from build123d import *

# Parameters (mm, degrees)
CROQUIS1_R                 = 2
SALIENTE_EXTRUIR1_DEPTH    = 16.65
CORTAR_EXTRUIR1_DEPTH      = 12.5
CORTAR_EXTRUIR1_DEPTH_BACK = 12.5
CROQUIS2_R                 = 2
CROQUIS2_R_2               = 1.505
REDONDEO1_R                = 0.5
REDONDEO2_R                = 0.5


with BuildPart() as part:
    # Croquis1 → Saliente-Extruir1 (new, symmetric)
    with BuildSketch(Plane(origin=(0, 0, 0), x_dir=(1, 0, 0), z_dir=(0, 1, 0))):
        with Locations(Location((0, 0, 0), (0, 0, 270))):
            Circle(CROQUIS1_R)
    extrude(amount=SALIENTE_EXTRUIR1_DEPTH, both=True)

    # Croquis2 → Cortar-Extruir1 (cut, two sides: drawn at the far end of the back side and taken through both)
    with BuildSketch(Plane(origin=(0, 0, 0), x_dir=(1, 0, 0), z_dir=(0, 1, 0)).offset(-CORTAR_EXTRUIR1_DEPTH_BACK)):
        with Locations(Location((0, 0, 0), (0, 0, 270))):
            Circle(CROQUIS2_R)
        with Locations(Location((0, 0, 0), (0, 0, 270))):
            Circle(CROQUIS2_R_2, mode=Mode.SUBTRACT)
    extrude(amount=CORTAR_EXTRUIR1_DEPTH + CORTAR_EXTRUIR1_DEPTH_BACK, mode=Mode.SUBTRACT)

    # Redondeo1
    # the kernel refuses this fillet: 0.5 mm, written as the material it adds along each edge
    with BuildSketch(Plane(origin=(0, -12.5, 0), x_dir=(0, 0, 1), z_dir=(-1, 0, 0))) as redondeo1_piece_1_section:
        with BuildLine():
            CenterArc((1.505 + REDONDEO1_R, REDONDEO1_R), REDONDEO1_R, 180, 90)
            Line((1.505, REDONDEO1_R), (1.505, 0))
            Line((1.505, 0), (1.505 + REDONDEO1_R, 0))
        make_face()
    redondeo1_piece_1 = revolve(axis=Axis((0, -12.5, 0), (0, 1, 0)), mode=Mode.PRIVATE)
    redondeo1_piece_1 = redondeo1_piece_1 & Plane(origin=(0, -12.357868044, 0), x_dir=(0, 0, 1), z_dir=(0, 1, 0)) * Cylinder(2, 9, mode=Mode.PRIVATE)
    add(redondeo1_piece_1)

    # Redondeo2
    # the kernel refuses this fillet: 0.5 mm, written as the material it adds along each edge
    with BuildSketch(Plane(origin=(0, 12.5, 0), x_dir=(0, 0, 1), z_dir=(-1, 0, 0))) as redondeo2_piece_1_section:
        with BuildLine():
            CenterArc((1.505 + REDONDEO2_R, -REDONDEO2_R), REDONDEO2_R, 90, 90)
            Line((1.505 + REDONDEO2_R, 0), (1.505, 0))
            Line((1.505, 0), (1.505, -REDONDEO2_R))
        make_face()
    redondeo2_piece_1 = revolve(axis=Axis((0, 12.5, 0), (0, 1, 0)), mode=Mode.PRIVATE)
    redondeo2_piece_1 = redondeo2_piece_1 & Plane(origin=(0, 12.357868044, 0), x_dir=(0, 0, 1), z_dir=(0, 1, 0)) * Cylinder(2, 9, mode=Mode.PRIVATE)
    add(redondeo2_piece_1)


solid = part.part
Source: CAD feature listing. Evaluate the final solid. Frame: model axes, mm. Coordinates: 2 decimals unless noted, no trailing zeros. Write each loop counter-clockwise with the first axis right and the second up, starting at its lowest first coordinate (ties: lowest second). Pieces come first, ordered by that corner, then holes. Notation, with made-up numbers: M 64,-28 L 115,-28 A29 ccw 115,0 Z; hole C -36.5,78 d10. An arc over 180 degrees is marked long. Use a Markdown table: item, result.
1) Section C-C, the plane y = 14.5. Output: boundary loops of the cut face in (x, z), then the cut area to 3 significant figures.
Conclusion:
| item | result |
|---|---|
| outline | C 0,0 d4 |
| area | 12.6 mm^2 |
2) Section A-A, the plane z = 0. Output: boundary loops of the cut face in (x, y) (3 decimals).
Conclusion:
| item | result |
|---|---|
| outline | M -2,-16.65 L 2,-16.65 L 2,-12.5 A0.5 cw 1.505,-12 L 1.505,12 A0.5 cw 2,12.5 L 2,16.65 L -2,16.65 L -2,12.5 A0.5 cw -1.505,12 L -1.505,-12 A0.5 cw -2,-12.5 Z |
3) Mould query, pull axis Y, two halves, no side actions, for faces 1 (the cylindrical face through (-2, 15, 0)), 2 (the cylindrical face through (-1.47, -0.17, -0.33)), 3 (the flat face through (0, 16.65, 0)). Classes: pulls with the +Y half, pulls with the -Y half, needs draft (parallel to the pull), parting line crosses it, or undercut.
Conclusion:
| item | result |
|---|---|
| face 1 | needs draft |
| face 2 | undercut |
| face 3 | pulls with the +Y half |
4) Ray query, L1, parallel to Y at x = 1.15, z = -1.6; L2, parallel to Y at x = -0.8, z = -1.5; L3, parallel to X at y = 1, z = 0.85. Return the intervals inside material, ascending.
Conclusion:
| item | result |
|---|---|
| L1 | y = -16.65 to -12.5, 12.5 to 16.65 |
| L2 | y = -16.65 to -12.4, 12.4 to 16.65 |
| L3 | x = -1.24 to 1.24 |
5) Section B-B, the plane x = 0. Output: boundary loops of the cut face in (y, z) (3 decimals).
Conclusion:
| item | result |
|---|---|
| outline | M -16.65,-2 L -12.5,-2 A0.5 cw -12,-1.505 L 12,-1.505 A0.5 cw 12.5,-2 L 16.65,-2 L 16.65,2 L 12.5,2 A0.5 cw 12,1.505 L -12,1.505 A0.5 cw -12.5,2 L -16.65,2 Z |
6) First-contact query: pin 1 Ø1 at (y, z) = (0, 1) entering from -X. Flat tip, straight axial feed; report the tip coordinate or a pass-through.
Conclusion:
| item | result |
|---|---|
| pin 1 | stops at x = -1.42 |
7) Section D-D, the plane y = 6. Output: boundary loops of the cut face in (x, z) (3 decimals), then the cut area to 3 significant figures.
Conclusion:
| item | result |
|---|---|
| outline | C 0,0 d3.01 |
| area | 7.12 mm^2 |
